Design review of the part built by this model. Coordinates are the model's own, in mm. A direction names the side the tool comes from. Give positions to 0.01 mm unless a question says otherwise; leave off trailing zeros. Loops run counter-clockwise (first coordinate to the right, second up) from the corner with the lowest first, then second, coordinate; pieces in that order, holes last.
from build123d import *

# Parameters (mm, degrees)
BOSS_EXTRUDE1_DEPTH = 22
CUT_EXTRUDE1_DEPTH  = 22


with BuildPart() as part:
    # Sketch1 → Boss-Extrude1 (new body)
    with BuildSketch(Plane.XY):
        with BuildLine():
            Line((6.75, 1.5), (6.75, 0))
            Line((6.75, 0), (1, 0))
            ThreePointArc((1, 0), (0.292893219, -0.292893219), (0, -1))
            Line((0, -1), (0, -45.5))
            ThreePointArc((0, -45.5), (0.292893219, -46.207106781), (1, -46.5))
            Line((1, -46.5), (24, -46.5))
            ThreePointArc((24, -46.5), (24.707106781, -46.207106781), (25, -45.5))
            Line((25, -45.5), (25, -1))
            ThreePointArc((25, -1), (24.707106781, -0.292893219), (24, 0))
            Line((24, 0), (18.25, 0))
            Line((18.25, 0), (18.25, 1.5))
            Line((18.25, 1.5), (6.75, 1.5))
        make_face()
    extrude(amount=BOSS_EXTRUDE1_DEPTH)

    # Sketch2 → Cut-Extrude1 (cut)
    with BuildSketch(Plane.XY.offset(22)):
        with BuildLine():
            Line((2, -1), (23, -1))
            ThreePointArc((23, -1), (23.707106781, -1.292893219), (24, -2))
            Line((24, -2), (24, -44.5))
            ThreePointArc((24, -44.5), (23.707106781, -45.207106781), (23, -45.5))
            Line((23, -45.5), (2, -45.5))
            ThreePointArc((2, -45.5), (1.292893219, -45.207106781), (1, -44.5))
            Line((1, -44.5), (1, -2))
            ThreePointArc((1, -2), (1.292893219, -1.292893219), (2, -1))
        make_face()
    extrude(amount=-CUT_EXTRUDE1_DEPTH, mode=Mode.SUBTRACT)


solid = part.part
Q1. Take a section at A-A (x = 3.25). Give the boundary of the cut face in (y, z).
Results:
outline: (-46.5, 0) - (-45.5, 0) - (-45.5, 22) - (-46.5, 22) - close; (-1, 0) - (0, 0) - (0, 22) - (-1, 22) - close
Q2. Tool access review of faces 5 (the face through (1.285, -1.301, 11.154)), 6 (the face through (24.699, -46.215, 10.846)), 7 (the face through (21, 0, 11)): name each direction out of +Z, -Z, +X, -X, +Y, -Y from which nothing blocks a thin tool from reaching the whole face with its end or side.
Results:
face 5: +Z, -Z
face 6: +Z, -Z, +X, -Y
face 7: +Z, -Z, +X, +Y
Q3. Take a section at C-C (z = 6). Give the boundary of the cut face in (x, y).
Results:
outline: (0, -45.5) arc R1 ccw to (1, -46.5) - (24, -46.5) arc R1 ccw to (25, -45.5) - (25, -1) arc R1 ccw to (24, 0) - (18.25, 0) - (18.25, 1.5) - (6.75, 1.5) - (6.75, 0) - (1, 0) arc R1 ccw to (0, -1) - close; hole (1, -44.5) arc R1 ccw to (2, -45.5) - (23, -45.5) arc R1 ccw to (24, -44.5) - (24, -2) arc R1 ccw to (23, -1) - (2, -1) arc R1 ccw to (1, -2) - close
Q4. Wall thickness on line 1 (X direction, y = -7.5, z = 6); line 2 (Y direction, x = 19.75, z = 19.5); line 3 (Y direction, x = 12.25, z = 14): over which ranges is each line inside the solid? List them lowest first.
Results:
line 1: x = 0 to 1, 24 to 25
line 2: y = -46.5 to -45.5, -1 to 0
line 3: y = -46.5 to -45.5, -1 to 1.5
Q5. Insertion check: pin 1 (3 mm diameter, centred on x = 21.5, z = 7.5, fed in from +Y); pin 2 (1.6 mm diameter, centred on y = 1, z = 6, fed in from -X). Each pin has a flat end and moves straight along its axis. Give the tip position at first contact, or say it passes through.
Results:
pin 1: stops at y = 0
pin 2: stops at x = 6.75
Q6. Draft analysis for pull direction Y (two halves, no side actions). For faces 1 (the face through (23.699, -1.285, 11.154)), 2 (the face through (24, -23, 11)), 3 (the face through (18.25, 1, 11)), 4 (the face through (4, 0, 11)), state which applies: pulls with the +Y half, pulls with the -Y half, needs draft (parallel to the pull), parting line crosses it, or undercut.
Results:
face 1: undercut
face 2: undercut
face 3: needs draft
face 4: pulls with the +Y half
Q7. Take a section at B-B (y = -16). Give the boundary of the cut face in (x, z).
Results:
outline: (0, 0) - (1, 0) - (1, 22) - (0, 22) - close; (24, 0) - (25, 0) - (25, 22) - (24, 22) - close
